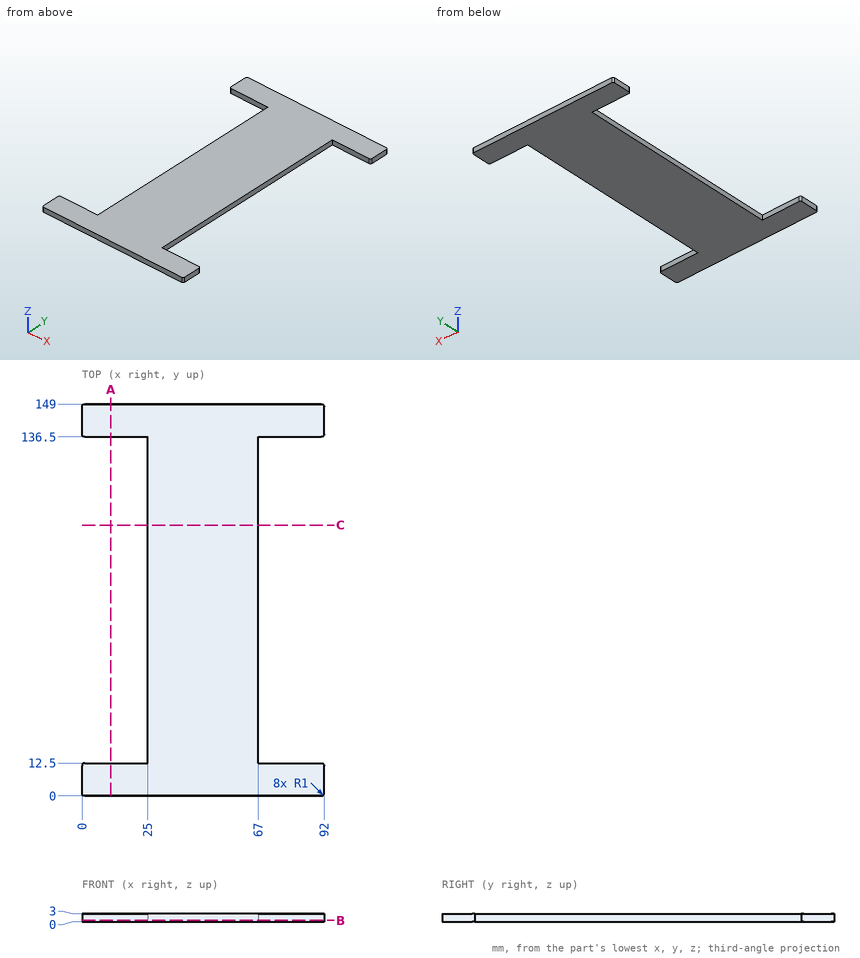
Geometry check sheet. Reference: drawing and pictorial views, mm from the part's lowest x, y, z. Round coordinates to 2 decimals unless told otherwise and drop trailing zeros. Write each loop counter-clockwise with the first axis right and the second up, starting at its lowest first coordinate (ties: lowest second). Pieces come first, ordered by that corner, then holes.
1. Section check A-A on x = 11. Enter the section's corners in (y, z).
2. Section check C-C on y = 103. Enter the section's corners in (x, z).
3. Gauge pin test, flat ends, axial feed: P1, Ø1.5, axis at y = 59, z = 1.5, coming from the -X side; P2, Ø1.5, axis at x = 23.5, y = 74.5, coming from the -Z side. Record the tip position at first contact, or that the pin passes through.
4. Section check B-B on z = 0.6. Enter the section's corners in (x, y).
5. Scan lines: L1, parallel to Y at x = 12.5, z = 2.6; L2, parallel to X at y = 20, z = 1.6. Record each from-to range of solid material in increasing order.
Answer:
1. outline: (0, 0) - (12.5, 0) - (12.5, 3) - (0, 3) - close; (136.5, 0) - (149, 0) - (149, 3) - (136.5, 3) - close
2. outline: (25, 0) - (67, 0) - (67, 3) - (25, 3) - close
3. P1: stops at x = 25
3. P2: passes through
4. outline: (0, 1) arc R1 ccw to (1, 0) - (91, 0) arc R1 ccw to (92, 1) - (92, 11.5) arc R1 ccw to (91, 12.5) - (67, 12.5) - (67, 136.5) - (91, 136.5) arc R1 ccw to (92, 137.5) - (92, 148) arc R1 ccw to (91, 149) - (1, 149) arc R1 ccw to (0, 148) - (0, 137.5) arc R1 ccw to (1, 136.5) - (25, 136.5) - (25, 12.5) - (1, 12.5) arc R1 ccw to (0, 11.5) - close
5. L1: y = 0 to 12.5, 136.5 to 149
5. L2: x = 25 to 67
